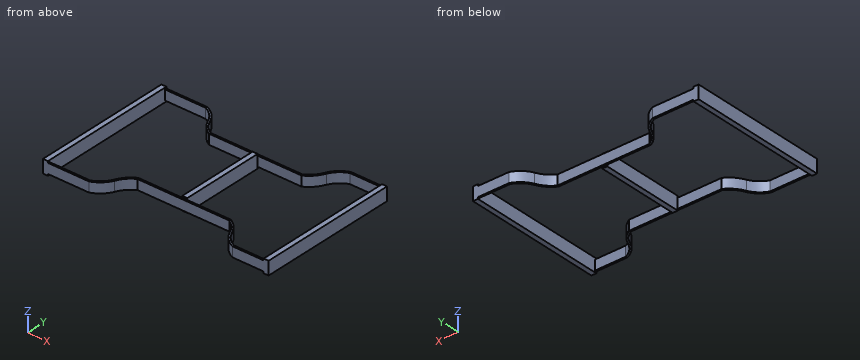
```python
from build123d import *

# Parameters (mm, degrees)
BOSS_EXTRUDE1_DEPTH   = 9.55
BOSS_EXTRUDE1_2_DEPTH = 9.55
SKETCH2_W             = 9.5
SKETCH2_H             = 266.7
SKETCH2_W_2           = 4.75
SKETCH2_H_2           = 158.7
BOSS_EXTRUDE2_DEPTH   = 12.7


with BuildPart() as part:
    # Sketch1 → Boss-Extrude1 (new, symmetric)
    with BuildSketch(Plane.XY):
        with BuildLine():
            Line((87.8, 266.7), (9.5, 266.7))
            Line((9.5, 266.7), (9.5, 263.5))
            Line((9.5, 263.5), (87.185653041, 263.5))
            ThreePointArc((87.185653041, 263.5), (101.872730764, 254.086326296), (112.181844193, 240.013313649))
            ThreePointArc((112.181844193, 240.013313649), (121.93402425, 224.242253512), (136.446354787, 212.7))
            Line((136.446354787, 212.7), (313.604913576, 212.7))
            ThreePointArc((313.604913576, 212.7), (328.117244113, 224.242253512), (337.86942417, 240.013313649))
            ThreePointArc((337.86942417, 240.013313649), (348.178537599, 254.086326296), (362.865615322, 263.5))
            Line((362.865615322, 263.5), (421.551268364, 263.5))
            Line((421.551268364, 263.5), (421.551268364, 266.7))
            Line((421.551268364, 266.7), (362.251268364, 266.7))
            ThreePointArc((362.251268364, 266.7), (346.178913489, 256.597493698), (334.937565202, 241.3))
            ThreePointArc((334.937565202, 241.3), (326.024834919, 226.70817797), (312.775634182, 215.9))
            Line((312.775634182, 215.9), (137.275634182, 215.9))
            ThreePointArc((137.275634182, 215.9), (124.026433444, 226.70817797), (115.113703162, 241.3))
            ThreePointArc((115.113703162, 241.3), (103.872354874, 256.597493698), (87.8, 266.7))
        make_face()
    extrude(amount=BOSS_EXTRUDE1_DEPTH, both=True)



with BuildPart() as body_2:
    # Sketch1 → Boss-Extrude1 2 (new, symmetric)
    with BuildSketch(Plane.XY):
        with BuildLine():
            Line((87.185653041, 3.2), (9.5, 3.2))
            Line((9.5, 3.2), (9.5, 0))
            Line((9.5, 0), (87.8, 0))
            ThreePointArc((87.8, 0), (103.872354874, 10.102506302), (115.113703162, 25.4))
            ThreePointArc((115.113703162, 25.4), (124.026433444, 39.99182203), (137.275634182, 50.8))
            Line((137.275634182, 50.8), (312.775634182, 50.8))
            ThreePointArc((312.775634182, 50.8), (326.024834919, 39.99182203), (334.937565202, 25.4))
            ThreePointArc((334.937565202, 25.4), (346.178913489, 10.102506302), (362.251268364, 0))
            Line((362.251268364, 0), (421.551268364, 0))
            Line((421.551268364, 0), (421.551268364, 3.2))
            Line((421.551268364, 3.2), (362.865615322, 3.2))
            ThreePointArc((362.865615322, 3.2), (348.178537599, 12.613673704), (337.86942417, 26.686686351))
            ThreePointArc((337.86942417, 26.686686351), (328.117244113, 42.457746488), (313.604913576, 54))
            Line((313.604913576, 54), (136.446354787, 54))
            ThreePointArc((136.446354787, 54), (121.93402425, 42.457746488), (112.181844193, 26.686686351))
            ThreePointArc((112.181844193, 26.686686351), (101.872730764, 12.613673704), (87.185653041, 3.2))
        make_face()
    extrude(amount=BOSS_EXTRUDE1_2_DEPTH, both=True)


with BuildPart() as part_1:
    add(part.part)

    add(body_2.part)  # Boss-Extrude2 merges body 2
    # Sketch2 → Boss-Extrude2 (add, symmetric)
    with BuildSketch(Plane.XY):
        with Locations((4.75, 133.35)):
            Rectangle(SKETCH2_W, SKETCH2_H)
        with Locations((222.650634182, 133.35)):
            Rectangle(SKETCH2_W_2, SKETCH2_H_2)
        with Locations((227.400634182, 133.35)):
            Rectangle(SKETCH2_W_2, SKETCH2_H_2)
        with Locations((426.301268364, 133.35)):
            Rectangle(SKETCH2_W, SKETCH2_H)
    extrude(amount=BOSS_EXTRUDE2_DEPTH, both=True)


solid = part_1.part
```
Geometry: final body of the model. Coordinates: model frame, mm. Coordinates: 2 decimals unless noted, no trailing zeros. Order: outer loops, then holes, each group sorted by start corner. A loop starts at its lowest first (then second) coordinate and runs counter-clockwise, first axis right, second up. Notation, with made-up numbers: (88, 33) -> (111, 33) arc R14 ccw to (111, 46) -> close; hole circle Ø5 at (-14, -24.75). An arc over 180 degrees is marked (long way). Answer in a Markdown table with one row per item.
Item 1: Ray query, L1, parallel to X at y = 68, z = 0.25; L2, parallel to Y at x = 86.5, z = -2; L3, parallel to Y at x = 295.5, z = -7. Return the intervals inside material, ascending.
Return value:
| item | result |
|---|---|
| L1 | x = 0 to 9.5, 220.28 to 229.78, 421.55 to 431.05 |
| L2 | y = 0 to 3.2, 263.5 to 266.7 |
| L3 | y = 50.8 to 54, 212.7 to 215.9 |
Item 2: Section A-A on x = 51. Output: boundary loops of the cut face in (y, z), plus the area to 3 significant figures.
Return value:
| item | result |
|---|---|
| outline | (0, -9.55) -> (3.2, -9.55) -> (3.2, 9.55) -> (0, 9.55) -> close; (263.5, -9.55) -> (266.7, -9.55) -> (266.7, 9.55) -> (263.5, 9.55) -> close |
| area | 122 mm² |
Item 3: Section B-B on y = 137. Output: boundary loops of the cut face in (x, z).
Return value:
| item | result |
|---|---|
| outline | (0, -12.7) -> (9.5, -12.7) -> (9.5, 12.7) -> (0, 12.7) -> close; (220.28, -12.7) -> (229.78, -12.7) -> (229.78, 12.7) -> (220.28, 12.7) -> close; (421.55, -12.7) -> (431.05, -12.7) -> (431.05, 12.7) -> (421.55, 12.7) -> close |
Item 4: Section D-D on x = 342. Output: boundary loops of the cut face in (y, z), plus the area to 3 significant figures.
Return value:
| item | result |
|---|---|
| outline | (14.48, -9.55) -> (19.69, -9.55) -> (19.69, 9.55) -> (14.48, 9.55) -> close; (247.01, -9.55) -> (252.22, -9.55) -> (252.22, 9.55) -> (247.01, 9.55) -> close |
| area | 199 mm² |
Item 5: Contact query for flat-ended pins moving along their axis: P1, Ø0.9, axis at x = 223, z = 11, coming from the -Y side; P2, Ø16, axis at x = 114.5, y = 253, coming from the +Z side; P3, Ø5.5, axis at x = 188, z = 4.5, coming from the +Y side. Output: stop coordinate, or through.
Return value:
| item | result |
|---|---|
| P1 | stops at y = 54 |
| P2 | stops at z = 9.55 |
| P3 | stops at y = 215.9 |
Item 6: Section C-C on z = -3.75. State how many separate pieces and enclosed holes the cut face has, plus the area to 3 significant figures.
Return value:
| item | result |
|---|---|
| separate pieces | 1 |
| enclosed holes | 2 |
| area | 9,510 mm² |
